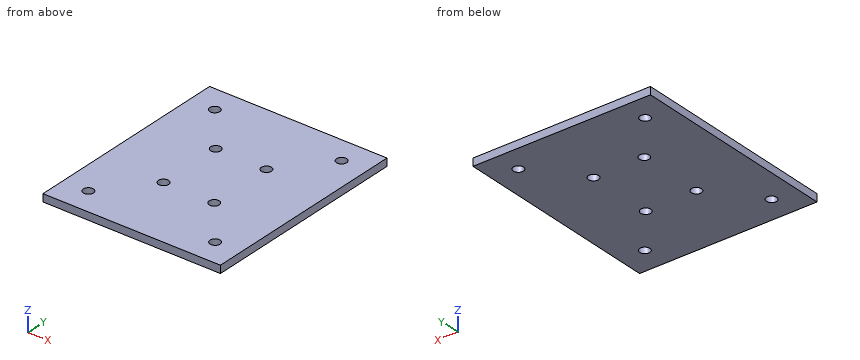
Autodesk Inventor part; units mm, degrees
ref_plane "YZ Plane" through (0, 0, 0) normal (1, 0, 0) x (0, 1, 0)
ref_plane "XZ Plane" through (0, 0, 0) normal (0, 1, 0) x (-1, 0, 0)
ref_plane "XY Plane" through (0, 0, 0) normal (0, 0, 1) x (1, 0, 0)
sketch "Sketch1" plane through (0, 0, 0) normal (0, 0, 1) x (1, 0, 0)
  line L0 (73, -75) -> (3, -75)
  line L1 (3, 8) -> (3, -75)
  line L2 (3, 8) -> (73, 8)
  line L3 (73, 8) -> (73, -75)
  circle A0 centre (13, -65) radius 2
  circle A1 centre (13, -2) radius 2
  circle A2 centre (63, -65) radius 2
  circle A3 centre (63, -2) radius 2
  circle A4 centre (28, -46.5) radius 2
  circle A5 centre (48, -46.5) radius 2
  line L4 (28, -46.5) -> (48, -46.5)
  circle A6 centre (28, -20.5) radius 2
  circle A7 centre (48, -20.5) radius 2
  line L5 (28, -20.5) -> (48, -20.5)
  point P0 (0, 0)
  dimension "d0" = 70
  dimension "d1" = 83
  dimension "d4" = 4
  dimension "d5" = 10
  dimension "d6" = 10
  dimension "d7" = 4
  dimension "d8" = 4
  dimension "d9" = 4
  dimension "d10" = 10
  dimension "d11" = 10
  dimension "d12" = 10
  dimension "d13" = 10
  dimension "d14" = 10
  dimension "d15" = 10
  dimension "d16" = 4
  dimension "d17" = 20
  dimension "d18" = 4
  dimension "d19" = 4
  dimension "d20" = 20
  dimension "d21" = 4
  dimension "d22" = 26
  dimension "d23" = 28.5
  dimension "d24" = 25
extrude "Extrusion1" add sketch "Sketch1" along normal blind 3
equation "\"d10\" = d5"
equation "\"d11\" = d6"
equation "\"d13\" = d12"
equation "\"d14\" = d13"
equation "\"d15\" = d14"
equation "\"d18\" = d16"
equation "\"d21\" = d19"
equation "\"d23\" = -0.5 * d22 + 0.5 * d1"
equation "\"d24\" = -0.5 * d17 + 0.5 * d0"
properties part number "BaseC_8" material "PMMA Plastic"
Verification items for the finished model (mm, model axes). Give positions to 0.01 mm unless a question says otherwise; leave off trailing zeros. Write each loop counter-clockwise with the first axis right and the second up, starting at its lowest first coordinate (ties: lowest second). Pieces come first, ordered by that corner, then holes.
(1) Cross-section at C-C (z = 0.55). State how many separate pieces and enclosed holes the cut face has, plus the area to 3 significant figures.
(2) Cross-section at A-A (x = 48). Enter the section's corners in (y, z).
(3) Cross-section at B-B (y = -20.5). Enter the section's corners in (x, z), plus the area to 3 significant figures.
(4) Material ranges on line 1 (Y direction, x = 28, z = 2.05); line 2 (Y direction, x = 63, z = 1.65); line 3 (X direction, y = -21.5, z = 1.1), recorded low to high.
Worked out:
1. separate pieces: 1
1. enclosed holes: 8
1. area: 5,710 mm2
2. outline: (-75, 0) - (-48.5, 0) - (-48.5, 3) - (-75, 3) - close; (-44.5, 0) - (-22.5, 0) - (-22.5, 3) - (-44.5, 3) - close; (-18.5, 0) - (8, 0) - (8, 3) - (-18.5, 3) - close
3. outline: (3, 0) - (26, 0) - (26, 3) - (3, 3) - close; (30, 0) - (46, 0) - (46, 3) - (30, 3) - close; (50, 0) - (73, 0) - (73, 3) - (50, 3) - close
3. area: 186 mm2
4. line 1: y = -75 to -48.5, -44.5 to -22.5, -18.5 to 8
4. line 2: y = -75 to -67, -63 to -4, 0 to 8
4. line 3: x = 3 to 26.27, 29.73 to 46.27, 49.73 to 73
